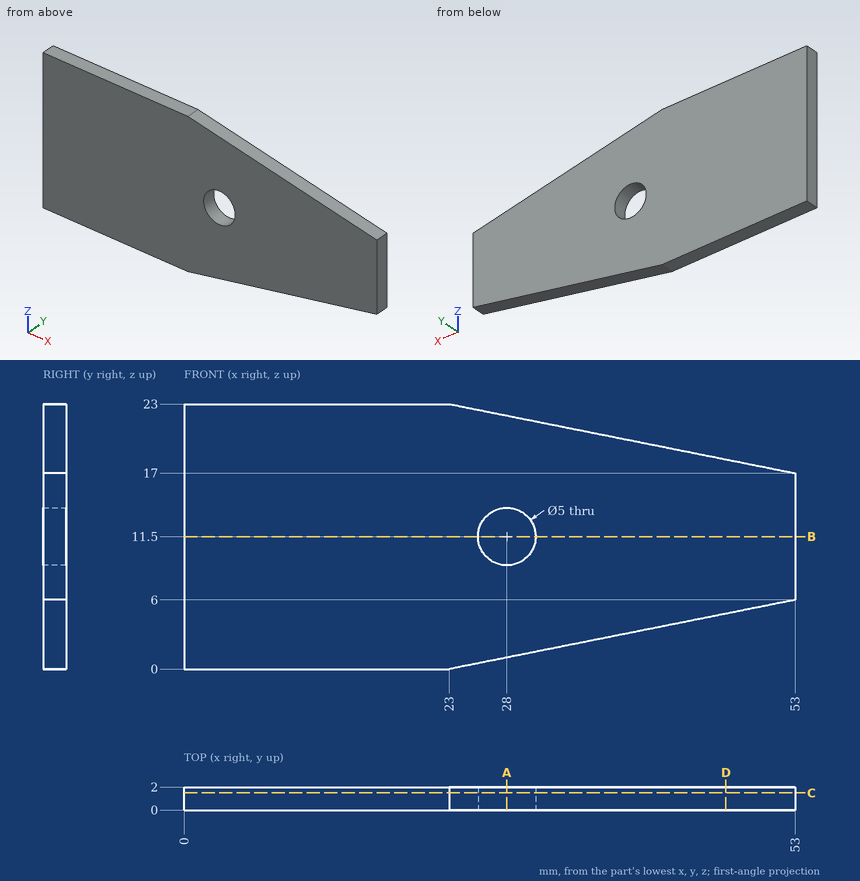
Input: dimensioned drawing with shaded views. Units: mm. Origin: part minimum x, y, z. Give positions to 0.01 mm unless a question says otherwise; leave off trailing zeros. Loops run counter-clockwise (first coordinate to the right, second up) from the corner with the lowest first, then second, coordinate; pieces in that order, holes last. Notation, with made-up numbers: M -20.75,14 L 11.25,14 A13 cw 11.25,20 Z; hole C 29.5,36 d8. An arc over 180 degrees is marked long. Put each result on its own line as item: value.
1) Cut plane C-C, the plane y = 1.5. Return the cut outline in (x, z), plus the area to 3 significant figures.
Computed values:
outline: M 0,0 L 23,0 L 53,6 L 53,17 L 23,23 L 0,23 Z; hole C 28,11.5 d5
area: 1,020 mm^2
2) Cut plane B-B, the plane z = 11.5. Return the cut outline in (x, y), plus the area to 3 significant figures.
Computed values:
outline: M 0,0 L 25.5,0 L 25.5,2 L 0,2 Z; M 30.5,0 L 53,0 L 53,2 L 30.5,2 Z
area: 96.0 mm^2
3) Cut plane D-D, the plane x = 47. Return the cut outline in (y, z).
Computed values:
outline: M 0,4.8 L 2,4.8 L 2,18.2 L 0,18.2 Z
4) Material intervals for L1, parallel to X at y = 0.75, z = 11.5; L2, parallel to X at y = 1.35, z = 10.5, sorted ascending. Write a range as from..to.
Computed values:
L1: x = 0..25.5, 30.5..53
L2: x = 0..25.71, 30.29..53
5) Cut plane A-A, the plane x = 28. Return the cut outline in (y, z).
Computed values:
outline: M 0,1 L 2,1 L 2,9 L 0,9 Z; M 0,14 L 2,14 L 2,22 L 0,22 Z
